Can you work these out from the model? Positions are in its coordinate system, mm. Coordinates: 2 decimals unless noted, no trailing zeros. Loops run counter-clockwise (first coordinate to the right, second up) from the corner with the lowest first, then second, coordinate; pieces in that order, holes last. Notation, with made-up numbers: M 33,21.25 L 44,21.25 A26 ccw 44,54.25 Z; hole C -22.75,52 d8. An arc over 180 degrees is marked long. Answer as a JSON object with one key per item and string values. Group by question number.
Item 1: If I drill on line 1 (X direction, y = -3, z = 5.25); line 2 (Y direction, x = -42, z = 16.25); line 3 (Y direction, x = -40, z = 17.5), over which ranges is the centre line in solid material (lowest first)?
Item 2: Suppose I cut it at A-A (z = 18.25). Write out the boundary of the cut face in (x, y).
Item 3: I'm going to push flat-ended pins straight in: pin 1 Ø1.5 at (x, z) = (-43, 6) entering from +Y; pin 2 Ø6 at (x, z) = (-35.5, 7.5) entering from +Y; pin 3 Ø10 at (y, z) = (-5.5, 10.5) entering from -X. Where does each tip first touch, or does it pass through?
```python
from build123d import *

# Parameters (mm, degrees)
F0_W     = 30
F0_H     = 30
F1_DEPTH = 25
F2_R     = 1


with BuildPart() as f1:
    # F0 (on Top) → F1 (new body)
    with BuildSketch(Plane.XY):
        with Locations((-9.894624, 1.663389)):
            Rectangle(F0_W, F0_H)
        Polygon((-24.894624, -13.336611), (-24.894624, 16.663389), (-54.894623, -13.327551), align=None)
    extrude(amount=F1_DEPTH)

    # F2
    f2_edges = [f1.edges().sort_by_distance(p)[0] for p in [
        (-39.894624, 1.667919, 25),
        (-39.894624, -13.332081, 25),
        (-9.894624, -13.336611, 25),
        (-9.894624, 16.663389, 25),
        (5.105376, 1.663389, 25),
        (-54.894623, -13.327551, 12.5),
        (-39.894624, -13.332081, 0),
        (-9.894624, -13.336611, 0),
        (5.105376, -13.336611, 12.5),
        (-24.894624, -13.336611, 12.5),
        (-39.894624, 1.667919, 0),
        (-24.894624, 16.663389, 12.5),
        (-9.894624, 16.663389, 0),
    ]]
    fillet(f2_edges, radius=F2_R)


solid = f1.part
```
From the geometry:
{
 "1": {"line 1": "-44.56 to 5.11", "line 2": "-13.33 to -0.44", "line 3": "-13.33 to 1.56"},
 "2": {"outline": "M -53.19,-11.62 A1 ccw -52.48,-13.33 L -24.89,-13.34 L 4.11,-13.34 A1 ccw 5.11,-12.34 L 5.11,16.66 L -24.48,16.66 A1 ccw -25.19,16.37 Z"},
 "3": {"pin 1": "y = -0.69", "pin 2": "y = 9.06", "pin 3": "x = -52.07"}
}
